```python
from build123d import *

# Parameters (mm, degrees)
F0_W         = 75.9326070547
F0_H         = 28.4124165773
F1_DEPTH     = 12.7
F2_W         = 24.4196355343
F2_H         = 12.4133229256
F3_DEPTH     = 177.8
F4_T1_DEPTH  = 53.8124165773
F4_T3_DEPTH  = 63.9811988592
F4_T5_DEPTH  = 190.5
F4_T10_DEPTH = 101.3326070547
F4_T16_DEPTH = 101.3326070547
F4_T22_DEPTH = 101.3326070547
F4_T29_DEPTH = 101.3326070547
F4_T35_DEPTH = 101.3326070547
F4_T42_DEPTH = 76.6811988592
F4_T46_DEPTH = 203.2
F5_R         = 5.08
F6_R         = 5.08


# Not quite as in the source:
# - a fillet or chamfer that OpenCascade refuses, or shapes differently, is made with other operations: its cross-section is extruded or revolved along the edge and cut away or added


with BuildPart() as f1:
    # F0 (on Top) → F1 (new body)
    with BuildSketch(Plane.XY):
        with Locations((-37.9663035274, 14.2062082887)):
            Rectangle(F0_W, F0_H)
    extrude(amount=F1_DEPTH)

    # F2 (on Front) → F3 (join)
    with BuildSketch(Plane.XZ):
        with Locations((-63.4910166264, 6.2066614628)):
            Rectangle(F2_W, F2_H)
    extrude(amount=F3_DEPTH)

    # F4: fillet of radius 5.08 on 5 edges, made by hand

    # F4_s2 → F4_t1 (cut)
    with BuildSketch(Plane.XZ.offset(-41.1124165773)):
        with BuildLine():
            ThreePointArc((-5.08, 0), (-1.4878975516, 1.4878975516), (0, 5.08))
            Line((0, 5.08), (0, 0))
            Line((0, 0), (-5.08, 0))
        make_face()
        with BuildLine():
            ThreePointArc((0, 7.62), (-1.4878975516, 11.2121024484), (-5.08, 12.7))
            Line((-5.08, 12.7), (0, 12.7))
            Line((0, 12.7), (0, 7.62))
        make_face()
    extrude(amount=F4_T1_DEPTH, mode=Mode.SUBTRACT)

    # F4_s4 → F4_t3 (cut)
    with BuildSketch(Plane.YZ.offset(-51.2811988592)):
        with BuildLine():
            ThreePointArc((0, 5.08), (1.4878975516, 1.4878975516), (5.08, 0))
            Line((5.08, 0), (0, 0))
            Line((0, 0), (0, 5.08))
        make_face()
    extrude(amount=F4_T3_DEPTH, mode=Mode.SUBTRACT)

    # F4_s6 → F4_t5 (cut)
    with BuildSketch(Plane.XZ):
        with BuildLine():
            ThreePointArc((-56.3611988592, 0), (-52.7690964108, 1.4878975516), (-51.2811988592, 5.08))
            Line((-51.2811988592, 5.08), (-51.2811988592, 0))
            Line((-51.2811988592, 0), (-56.3611988592, 0))
        make_face()
    extrude(amount=F4_T5_DEPTH, mode=Mode.SUBTRACT)


with BuildPart() as f4_tool8:
    # F4_s9 → F4_t10 (new body)
    with BuildSketch(Plane.YZ.offset(-88.6326070547)):
        with BuildLine():
            ThreePointArc((0, 7.62), (1.4878975516, 11.2121024484), (5.08, 12.7))
            Line((5.08, 12.7), (0, 12.7))
            Line((0, 12.7), (0, 7.62))
        make_face()
    extrude(amount=F4_T10_DEPTH)

    split(bisect_by=Plane.YZ.offset(-75.7008343935), keep=Keep.BOTTOM)

    split(bisect_by=Plane.XY.offset(12.4133229256), keep=Keep.BOTTOM)


with BuildPart() as f1_1:
    add(f1.part)

    # F4_t7: cut F4_tool8
    add(f4_tool8.part, mode=Mode.SUBTRACT)


with BuildPart() as f4_tool14:
    # F4_s15 → F4_t16 (new body)
    with BuildSketch(Plane.YZ.offset(-88.6326070547)):
        with BuildLine():
            ThreePointArc((0, 7.62), (1.4878975516, 11.2121024484), (5.08, 12.7))
            Line((5.08, 12.7), (0, 12.7))
            Line((0, 12.7), (0, 7.62))
        make_face()
    extrude(amount=F4_T16_DEPTH)

    split(bisect_by=Plane.YZ.offset(-75.7008343935), keep=Keep.BOTTOM)

    split(bisect_by=Plane.XY.offset(12.4133229256), keep=Keep.TOP)


with BuildPart() as f1_2:
    add(f1_1.part)

    # F4_t13: cut F4_tool14
    add(f4_tool14.part, mode=Mode.SUBTRACT)


with BuildPart() as f4_tool20:
    # F4_s21 → F4_t22 (new body)
    with BuildSketch(Plane.YZ.offset(-88.6326070547)):
        with BuildLine():
            ThreePointArc((0, 7.62), (1.4878975516, 11.2121024484), (5.08, 12.7))
            Line((5.08, 12.7), (0, 12.7))
            Line((0, 12.7), (0, 7.62))
        make_face()
    extrude(amount=F4_T22_DEPTH)

    split(bisect_by=Plane.YZ.offset(-75.7008343935), keep=Keep.TOP)

    split(bisect_by=Plane.XY.offset(12.4133229256), keep=Keep.TOP)

    split(bisect_by=Plane.YZ.offset(-51.2811988592), keep=Keep.BOTTOM)


with BuildPart() as f1_3:
    add(f1_2.part)

    # F4_t19: cut F4_tool20
    add(f4_tool20.part, mode=Mode.SUBTRACT)


with BuildPart() as f4_tool27:
    # F4_s28 → F4_t29 (new body)
    with BuildSketch(Plane.YZ.offset(-88.6326070547)):
        with BuildLine():
            ThreePointArc((0, 7.62), (1.4878975516, 11.2121024484), (5.08, 12.7))
            Line((5.08, 12.7), (0, 12.7))
            Line((0, 12.7), (0, 7.62))
        make_face()
    extrude(amount=F4_T29_DEPTH)

    split(bisect_by=Plane.XY.offset(12.4133229256), keep=Keep.BOTTOM)

    split(bisect_by=Plane.YZ.offset(-51.2811988592), keep=Keep.TOP)


with BuildPart() as f1_4:
    add(f1_3.part)

    # F4_t26: cut F4_tool27
    add(f4_tool27.part, mode=Mode.SUBTRACT)


with BuildPart() as f4_tool33:
    # F4_s34 → F4_t35 (new body)
    with BuildSketch(Plane.YZ.offset(-88.6326070547)):
        with BuildLine():
            ThreePointArc((0, 7.62), (1.4878975516, 11.2121024484), (5.08, 12.7))
            Line((5.08, 12.7), (0, 12.7))
            Line((0, 12.7), (0, 7.62))
        make_face()
    extrude(amount=F4_T35_DEPTH)

    split(bisect_by=Plane.XY.offset(12.4133229256), keep=Keep.TOP)

    split(bisect_by=Plane.YZ.offset(-51.2811988592), keep=Keep.TOP)


with BuildPart() as f1_5:
    add(f1_4.part)

    # F4_t32: cut F4_tool33
    add(f4_tool33.part, mode=Mode.SUBTRACT)


with BuildPart() as f4_tool40:
    # F4_s41 → F4_t42 (new body)
    with BuildSketch(Plane.YZ.offset(-63.9811988592)):
        with BuildLine():
            ThreePointArc((0, 5.08), (1.4878975516, 1.4878975516), (5.08, 0))
            Line((5.08, 0), (0, 0))
            Line((0, 0), (0, 5.08))
        make_face()
    extrude(amount=F4_T42_DEPTH)

    split(bisect_by=Plane.YZ.offset(-51.2811988592), keep=Keep.BOTTOM)


with BuildPart() as f4_tool44:
    # F4_s45 → F4_t46 (new body)
    with BuildSketch(Plane.XZ.offset(-12.7)):
        with BuildLine():
            ThreePointArc((-56.3611988592, 0), (-52.7690964108, 1.4878975516), (-51.2811988592, 5.08))
            Line((-51.2811988592, 5.08), (-51.2811988592, 0))
            Line((-51.2811988592, 0), (-56.3611988592, 0))
        make_face()
    extrude(amount=F4_T46_DEPTH)

    split(bisect_by=Plane.XZ, keep=Keep.BOTTOM)


with BuildPart() as f4_tool40_1:
    add(f4_tool40.part)

    # F4_t48: intersect F4_tool44
    add(f4_tool44.part, mode=Mode.INTERSECT)


with BuildPart() as f1_6:
    add(f1_5.part)

    # F4_t38: cut F4_tool40
    add(f4_tool40_1.part, mode=Mode.SUBTRACT)

    # F5
    f5_edges = [f1_6.edges().sort_by_distance(p)[0] for p in [
        (-51.281199, -87.201198, 12.413323),
        (-75.700834, -87.201198, 12.413323),
        (-75.700834, -88.9, 0),
    ]]
    fillet(f5_edges, radius=F5_R)

    # F6
    f6_edges = [f1_6.edges().sort_by_distance(p)[0] for p in [
        (-75.932607, 14.206208, 0),
        (-75.932607, 28.412417, 6.35),
        (-40.506304, 28.412417, 0),
    ]]
    fillet(f6_edges, radius=F6_R)


solid = f1_6.part
```
Geometry check sheet. Reference: the model listing, model coordinates, mm. A direction names the side the tool comes from. Round coordinates to 2 decimals unless told otherwise and drop trailing zeros. Loops run counter-clockwise (first coordinate to the right, second up) from the corner with the lowest first, then second, coordinate; pieces in that order, holes last. Notation, with made-up numbers: (38.25, 12.5) - (95.25, 12.5) arc R16 ccw to (95.25, 24.5) - close; hole circle Ø3 at (52.5, 43). An arc over 180 degrees is marked (long way). Use a Markdown table: item, result.
Q1. Go/stop test with flat-tipped pins: P1, Ø1.5, axis at y = -89.5, z = 6.5, coming from the -X side; P2, Ø1.8, axis at y = -96.5, z = 6.5, coming from the +X side; P3, Ø1, axis at y = -123.5, z = 1.5, coming from the -X side. Record where each tip stops, or that it passes through.
Solutions:
| item | result |
|---|---|
| P1 | stops at x = -75.7 |
| P2 | stops at x = -51.28 |
| P3 | stops at x = -74.66 |
Q2. Cross-section at D-D on x = -53.5. Record the cut outline in (y, z), plus the area to 3 significant figures.
Solutions:
| item | result |
|---|---|
| outline | (-177.8, 0.88) - (2.22, 0.88) arc R5.08 ccw to (5.08, 0) - (23.33, 0) arc R5.08 ccw to (28.41, 5.08) - (28.41, 7.62) arc R5.08 ccw to (23.33, 12.7) - (5.08, 12.7) arc R5.08 ccw to (1.84, 11.53) - (-177.8, 11.53) - close |
| area | 2,240 mm2 |
Q3. Cross-section at A-A on x = -11.5. Record the cut outline in (y, z), plus the area to 3 significant figures.
Solutions:
| item | result |
|---|---|
| outline | (0, 5.08) arc R5.08 ccw to (5.08, 0) - (23.33, 0) arc R5.08 ccw to (28.41, 5.08) - (28.41, 7.62) arc R5.08 ccw to (23.33, 12.7) - (5.08, 12.7) arc R5.08 ccw to (0, 7.62) - close |
| area | 339 mm2 |
Q4. Cross-section at B-B on y = -30. Record the cut outline in (x, z), plus the area to 3 significant figures.
Solutions:
| item | result |
|---|---|
| outline | (-75.7, 5.08) arc R5.08 ccw to (-70.62, 0) - (-56.36, 0) arc R5.08 ccw to (-51.28, 5.08) - (-51.28, 7.33) arc R5.08 ccw to (-56.36, 12.41) - (-70.62, 12.41) arc R5.08 ccw to (-75.7, 7.33) - close |
| area | 281 mm2 |
Q5. Cross-section at C-C on z = 2.5. Record the cut outline in (x, y), plus the area to 3 significant figures.
Solutions:
| item | result |
|---|---|
| outline | (-75.23, 0) - (-75, 0) - (-75, -177.8) - (-51.99, -177.8) - (-51.99, 0.7) - (-0.7, 0.7) - (-0.7, 23.33) arc R4.38 ccw to (-5.08, 27.71) - (-70.85, 27.71) arc R4.38 ccw to (-75.23, 23.33) - close |
| area | 6,110 mm2 |
Q6. Material ranges on line 1 (X direction, y = -28, z = 7.75); line 2 (X direction, y = 14, z = 7.75); line 3 (Z direction, x = -59.5, y = -19), recorded low to high.
Solutions:
| item | result |
|---|---|
| line 1 | x = -75.68 to -51.3 |
| line 2 | x = -75.93 to 0 |
| line 3 | z = 0 to 12.41 |
Q7. Access from +Z, -Z, +X, -X, +Y, -Y to the whole of each face (thin tool, end or side, straight path). Record for faces 1 (the flat face through (-64, -86, 12.413)), 2 (the cylindrical face through (-52.73, -85.933, 10.886)), 3 (the cylindrical face through (-74.173, -85.933, 10.965)), 4 (the cylindrical face through (-74.252, -90.145, 1.528)), 5 (the cylindrical face through (-52.81, -85.08, 1.45)).
Solutions:
| item | result |
|---|---|
| face 1 | +Z, +X, -X, -Y |
| face 2 | +Z, +X, -Y |
| face 3 | +Z, -X, -Y |
| face 4 | -Z, -X, -Y |
| face 5 | -Z, +X, -Y |
